The listing builds one solid part. Answer for the finished solid, in the listing's coordinates (mm). Face numbers are marked on the shaded views. A direction names the side the tool comes from. Coordinates: 2 decimals unless noted, no trailing zeros. Write each loop counter-clockwise with the first axis right and the second up, starting at its lowest first coordinate (ties: lowest second). Pieces come first, ordered by that corner, then holes.
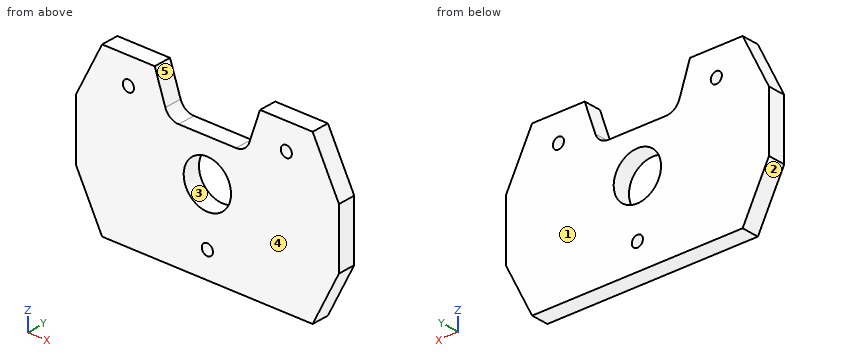
from build123d import *

# Parameters (mm, degrees)
SKETCH1_R           = 3.175
SKETCH1_R_2         = 13.5
BOSS_EXTRUDE1_DEPTH = 10


with BuildPart() as part:
    # Sketch1 → Boss-Extrude1 (new body)
    with BuildSketch(Plane(origin=(0, 0, 0), x_dir=(1, 0, 0), z_dir=(0, 1, 0))):
        with BuildLine():
            Line((-60, 27.300970874), (60, 27.300970874))
            Line((60, 27.300970874), (75, -2.699029126))
            Line((75, -2.699029126), (75, -36.699029126))
            Line((75, -36.699029126), (60, -66.699029126))
            Line((60, -66.699029126), (30, -66.699029126))
            Line((30, -66.699029126), (23.949215607, -48.655488788))
            ThreePointArc((23.949215607, -48.655488788), (21.036148951, -44.704865488), (16.364335743, -43.199029126))
            Line((16.364335743, -43.199029126), (-16.364335743, -43.199029126))
            ThreePointArc((-16.364335743, -43.199029126), (-21.036148951, -44.704865488), (-23.949215607, -48.655488788))
            Line((-23.949215607, -48.655488788), (-30, -66.699029126))
            Line((-30, -66.699029126), (-60, -66.699029126))
            Line((-60, -66.699029126), (-75, -36.699029126))
            Line((-75, -36.699029126), (-75, -2.699029126))
            Line((-75, -2.699029126), (-60, 27.300970874))
        make_face()
        with Locations(Location((-45, -51.699029126, 0), (0, 0, 270))):
            Circle(SKETCH1_R, mode=Mode.SUBTRACT)
        with Locations(Location((0, 12.300970874, 0), (0, 0, 270))):
            Circle(SKETCH1_R, mode=Mode.SUBTRACT)
        with Locations(Location((45, -51.699029126, 0), (0, 0, 270))):
            Circle(SKETCH1_R, mode=Mode.SUBTRACT)
        with Locations(Location((0, -19.699029126, 0), (0, 0, 270))):
            Circle(SKETCH1_R_2, mode=Mode.SUBTRACT)
    extrude(amount=BOSS_EXTRUDE1_DEPTH)


solid = part.part
Q1. The part is cut by section A-A, the plane z = 28.5. Write down the section's boundary in (x, y).
Answers below:
outline: (-75, 0) - (-10.24, 0) - (-10.24, 10) - (-75, 10) - close; (10.24, 0) - (75, 0) - (75, 10) - (10.24, 10) - close
Q2. Find the intervals of material crossed by probe 1 along X at (y, z) = (8.25, 23); probe 2 along X at (y, z) = (4, 8); probe 3 along X at (y, z) = (1.25, -21), in increasing order.
Answers below:
probe 1: x = -75 to -13.09, 13.09 to 75
probe 2: x = -75 to -6.74, 6.74 to 75
probe 3: x = -63.15 to 63.15
Q3. The part is cut by section C-C, the plane x = -45. Write down the section's boundary in (y, z).
Answers below:
outline: (0, -27.3) - (10, -27.3) - (10, 48.52) - (0, 48.52) - close; (0, 54.87) - (10, 54.87) - (10, 66.7) - (0, 66.7) - close
Q4. The part is cut by section D-D, the plane x = 0. Write down the section's boundary in (y, z).
Answers below:
outline: (0, -27.3) - (10, -27.3) - (10, -15.48) - (0, -15.48) - close; (0, -9.13) - (10, -9.13) - (10, 6.2) - (0, 6.2) - close; (0, 33.2) - (10, 33.2) - (10, 43.2) - (0, 43.2) - close
Q5. Determine the mould class of the marked faces 1, 2 and 3 for opening direction X: released by +X, released by -X, zero draft, split by the parting line, or undercut.
Answers below:
face 1: zero draft
face 2: released by -X
face 3: undercut
Q6. Which of the six approach directions +Z, -Z, +X, -X, +Y, -Y give full straight-line access (tool end or side, diameter ignored) to the marked faces 4 and 5?
Answers below:
face 4: +Z, -Z, +X, -X, -Y
face 5: +Z, +Y, -Y
Q7. Given pin 1 (12 mm diameter, centred on x = -44, z = 50, fed in from -Y); pin 2 (3 mm diameter, centred on x = -4, y = 4.5, fed in from +Z); pin 3 (5 mm diameter, centred on x = -45, z = 51.7, fed in from +Y); pin 4 (2 mm diameter, centred on y = 2.5, z = 53, fed in from +X), each flat-ended and moving along its own axis, determine where each tip first touches the part or whether it passes through.
Answers below:
pin 1: stops at y = 0
pin 2: stops at z = 43.2
pin 3: passes through
pin 4: stops at x = 67.35
Q8. The part is cut by section B-B, the plane y = 7.25. Write down the section's boundary in (x, z) (3 decimals).
Answers below:
outline: (-75, 2.699) - (-60, -27.301) - (60, -27.301) - (75, 2.699) - (75, 36.699) - (60, 66.699) - (30, 66.699) - (23.949, 48.655) arc R8 cw to (16.364, 43.199) - (-16.364, 43.199) arc R8 cw to (-23.949, 48.655) - (-30, 66.699) - (-60, 66.699) - (-75, 36.699) - close; hole circle Ø6.35 at (-45, 51.699); hole circle Ø27 at (0, 19.699); hole circle Ø6.35 at (0, -12.301); hole circle Ø6.35 at (45, 51.699)
